Input: part model. Units: mm. Frame: model coordinates. A direction names the side the tool comes from. Coordinates: 2 decimals unless noted, no trailing zeros. Write each loop counter-clockwise with the first axis right and the second up, starting at its lowest first coordinate (ties: lowest second). Pieces come first, ordered by that corner, then holes. Notation, with made-up numbers: (-29.75, 5.25) - (-20.75, 5.25) arc R20 ccw to (-20.75, 23.25) - close; hole circle Ø9 at (57.25, 86.5). An arc over 180 degrees is marked (long way). Use a Markdown table: item, result. Add a question column.
Q1. Section query A-A (y = -31). Return the cut outline in (x, z).
Q2. Material intervals for probe 1 along X at (y, z) = (-16, -32); probe 2 along Z at (x, y) = (3.5, -19); probe 3 along Y at (x, z) = (-17.5, -8), sorted ascending. Write a range as from..to.
Q3. Section query C-C (z = 9). Return the cut outline in (x, y), then the cut area to 3 significant figures.
Q4. Mould query, pull axis X, two halves, no side actions, for faces 1 (the face through (-17.47, -7.6, 14.69)), 2 (the face through (-29.15, -7.4, 31.84)), 3 (the face through (13.246, -20, -29)), 4 (the face through (-7, 0, 2)). Classes: released by +X, released by -X, zero draft, split by the parting line, or undercut.
Q5. Section query B-B (x = -12). Return the cut outline in (y, z).
Q6. Set-up query: faces 5 (the face through (-7, -40, -21)), 6 (the face through (-6, -27, -11.813)), 7 (the face through (-26.754, -20, -29)). Return all of +Z, -Z, +X, -X, +Y, -Y with unobstructed straight access to the full face (end or side cutting, diameter ignored); none if empty.
Q7. Pin query (flat end, axial travel): P1, Ø20, axis at x = 2, y = -25, coming from the -Z side; P2, Ø20, axis at x = -4, y = -29, coming from the +Z side; P3, Ø15.5, axis at x = -14.5, z = 5, coming from the -Y side. Return the tip coordinate at first contact, or that it passes through.
Q8. Section query D-D (x = 19). Return the cut outline in (y, z), then the cut area to 3 significant figures.
from build123d import *

# Parameters (mm, degrees)
F1_DEPTH = 15
F3_DEPTH = 25
F4_R     = 10.019997
F5_DEPTH = 25


with BuildPart() as f1:
    # F0 (on Front) → F1 (new body)
    with BuildSketch(Plane.XZ):
        Polygon((-21.754347, 39.233197), (-36.754347, 24.233197), (-36.754347, -35.766803), (-26.754347, -35.766803), (-26.754347, -22.329369), (13.245653, -22.329369), (13.245653, -35.766803), (23.245653, -35.766803), (23.245653, 39.233197), align=None)
    extrude(amount=F1_DEPTH)

    # F2 (on face) → F3 (join)
    with BuildSketch(Plane.XZ.offset(15)):
        Polygon((23.245653, -11.812501), (-36.754347, -11.812501), (-36.754347, -35.766803), (-26.754347, -35.766803), (-26.754347, -22.329369), (13.245653, -22.329369), (13.245653, -35.766803), (23.245653, -35.766803), align=None)
    extrude(amount=F3_DEPTH)

    # F4 (on face) → F5 (cut)
    with BuildSketch(Plane.XZ.offset(15)):
        with Locations((-7.458407, 14.252321)):
            Circle(F4_R)
    extrude(amount=-F5_DEPTH, mode=Mode.SUBTRACT)


solid = f1.part
Values follow:
| question | item | result |
|---|---|---|
| 1 | outline | (-36.75, -35.77) - (-26.75, -35.77) - (-26.75, -22.33) - (13.25, -22.33) - (13.25, -35.77) - (23.25, -35.77) - (23.25, -11.81) - (-36.75, -11.81) - close |
| 2 | probe 1 | -36.75..-26.75, 13.25..23.25 |
| 2 | probe 2 | -22.33..-11.81 |
| 2 | probe 3 | -15..0 |
| 3 | outline | (-36.75, -15) - (-15.99, -15) - (-15.99, 0) - (-36.75, 0) - close; (1.07, -15) - (23.25, -15) - (23.25, 0) - (1.07, 0) - close |
| 3 | area | 644 mm2 |
| 4 | face 1 | undercut |
| 4 | face 2 | released by -X |
| 4 | face 3 | undercut |
| 4 | face 4 | zero draft |
| 5 | outline | (-40, -22.33) - (0, -22.33) - (0, 5.32) - (-15, 5.32) - (-15, -11.81) - (-40, -11.81) - close; (-15, 23.18) - (0, 23.18) - (0, 39.23) - (-15, 39.23) - close |
| 6 | face 5 | +Z, -Z, +X, -X, -Y |
| 6 | face 6 | +Z, +X, -X, -Y |
| 6 | face 7 | -Z, +Y, -Y |
| 7 | P1 | z = -22.33 |
| 7 | P2 | z = -11.81 |
| 7 | P3 | y = -15 |
| 8 | outline | (-40, -35.77) - (0, -35.77) - (0, 39.23) - (-15, 39.23) - (-15, -11.81) - (-40, -11.81) - close |
| 8 | area | 1,720 mm2 |
